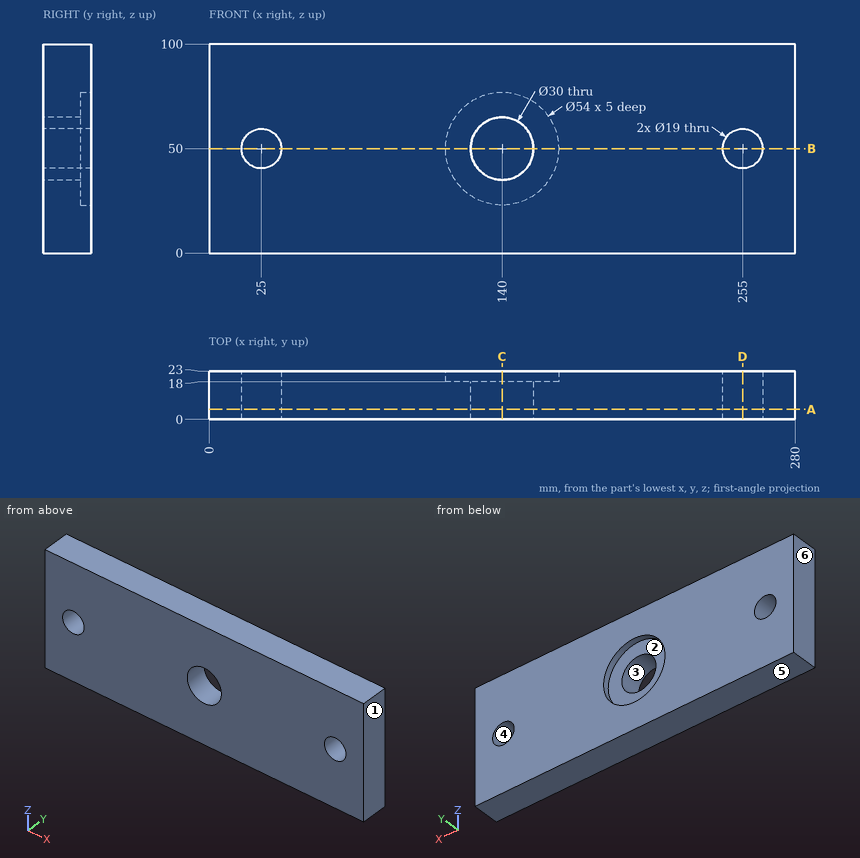
The drawing under review shows one solid part. Ordinate dimensions are in mm from its lowest x, y, z. A direction names the side the tool comes from. Coordinates: 2 decimals unless noted, no trailing zeros. Order: outer loops, then holes, each group sorted by start corner. A loop starts at its lowest first (then second) coordinate and runs counter-clockwise, first axis right, second up. Notation, with made-up numbers: (-20.75, 89.5) -> (35.25, 89.5) arc R27 ccw to (35.25, 128.5) -> close; hole circle Ø3 at (-38, 28.25). An arc over 180 degrees is marked (long way). Answer in a Markdown table with one row per item.
(1) Insertion check: pin 1 (3 mm diameter, centred on x = 43.5, y = 9.5, fed in from -Z). The pin has a flat end and moves straight along its axis. Give the tip position at first contact, or say it passes through.
Answers:
| item | result |
|---|---|
| pin 1 | z = 0 |
(2) Consider section D-D (x = 255). Write out the cut boundary in (y, z).
Answers:
| item | result |
|---|---|
| outline | (0, 0) -> (23, 0) -> (23, 40.5) -> (0, 40.5) -> close; (0, 59.5) -> (23, 59.5) -> (23, 100) -> (0, 100) -> close |
(3) The part is to be moulded in two halves that separate along X. For the marked faces 3, 4, 5 and 6, say which applies: +X half, -X half, draft (parallel to the pull), parting line (faces both ways), or undercut.
Answers:
| item | result |
|---|---|
| face 3 | undercut |
| face 4 | undercut |
| face 5 | draft |
| face 6 | -X half |
(4) Consider section B-B (z = 50). Write out the cut boundary in (x, y).
Answers:
| item | result |
|---|---|
| outline | (0, 0) -> (15.5, 0) -> (15.5, 23) -> (0, 23) -> close; (34.5, 0) -> (125, 0) -> (125, 18) -> (113, 18) -> (113, 23) -> (34.5, 23) -> close; (155, 0) -> (245.5, 0) -> (245.5, 23) -> (167, 23) -> (167, 18) -> (155, 18) -> close; (264.5, 0) -> (280, 0) -> (280, 23) -> (264.5, 23) -> close |
(5) Consider section C-C (x = 140). Write out the cut boundary in (y, z).
Answers:
| item | result |
|---|---|
| outline | (0, 0) -> (23, 0) -> (23, 23) -> (18, 23) -> (18, 35) -> (0, 35) -> close; (0, 65) -> (18, 65) -> (18, 77) -> (23, 77) -> (23, 100) -> (0, 100) -> close |
(6) Wall thickness on line 1 along X through (y, z) = (20.75, 49.5); line 2 along Z through (x, y) = (25, 6.25); line 3 along X through (y, z) = (19, 48): over which ranges is each line inside the solid? List them lowest first.
Answers:
| item | result |
|---|---|
| line 1 | 0 to 15.51, 34.49 to 113, 167 to 245.51, 264.49 to 280 |
| line 2 | 0 to 40.5, 59.5 to 100 |
| line 3 | 0 to 15.71, 34.29 to 113.07, 166.93 to 245.71, 264.29 to 280 |
(7) Consider section A-A (y = 4.75). Write out the cut boundary in (x, z), plus the area to 3 significant figures.
Answers:
| item | result |
|---|---|
| outline | (0, 0) -> (280, 0) -> (280, 100) -> (0, 100) -> close; hole circle Ø19 at (25, 50); hole circle Ø30 at (140, 50); hole circle Ø19 at (255, 50) |
| area | 26,700 mm² |
(8) Machinability: for the marked faces 1 and 2, which of the approach directions +Z, -Z, +X, -X, +Y, -Y give a long, thin tool a straight path to every point of the face, cutting with its end or side? Answer none if there is none.
Answers:
| item | result |
|---|---|
| face 1 | +Z, -Z, +X, +Y, -Y |
| face 2 | +Y |
